Work out the finished part from the listing and answer in its coordinate system (mm). A direction names the side the tool comes from. Give positions to 0.01 mm unless a question says otherwise; leave off trailing zeros. Write each loop counter-clockwise with the first axis right and the second up, starting at its lowest first coordinate (ties: lowest second). Pieces come first, ordered by that corner, then holes.
1) Find section A-A (z = 43.5). Determine the outline of the cut face in (x, y).
2) Straight lines are drawn through the part: probe 1 along Y at (x, z) = (6.5, 62.5); probe 2 along Z at (x, y) = (12, 43); probe 3 along X at (y, z) = (4, 28.5). For each, find the intervals that lie inside material, in ascending order.
3) Find section B-B (y = 3.5). Determine the outline of the cut face in (x, z), plus the area to 3 significant figures.
4) Find section C-C (z = 30). Determine the outline of the cut face in (x, y).
5) Given pin 1 Ø1 at (x, z) = (-15, 25.5) entering from +Y; pin 2 Ø1 at (y, z) = (49.5, 27.5) entering from +X; pin 3 Ø1.1 at (y, z) = (48, 24) entering from +X, each flat-ended and moving along its own axis, determine where each tip first touches the part or whether it passes through.
6) A tool of negligible diameter and unlimited length cuts with its end or side. For faces 1 (the face through (62.568, 25, 32)), 2 (the face through (34, 15, 2)), 3 (the face through (-40, 36.036, 32)), 4 (the face through (11, 8, 62.296)), from which of +Z, -Z, +X, -X, +Y, -Y can it reach the whole face along a straight path? Write none if from no direction.
7) Find section D-D (x = 23). Determine the outline of the cut face in (y, z).
8) Determine the mould class of faces 5 (the face through (-40, 39, 37.296)), 6 (the face through (10, 25, 0.296)), 7 (the face through (34, 47.4, 2)), 8 (the face through (10, 2, 32)) for opening direction Y: pulls with the +Y half, pulls with the -Y half, needs draft (parallel to the pull), parting line crosses it, or undercut.
Autodesk Fusion 360 part; units mm, degrees
sketch "Esquisse1" plane through (0, 0, 0) normal (0, 1, 0) x (1, 0, 0)
  line L0 (-41.4317, -0.2961) -> (62.5683, -0.2961)
  line L1 (62.5683, -0.2961) -> (62.5683, -64.2961)
  line L2 (62.5683, -64.2961) -> (-41.4317, -64.2961)
  line L3 (-41.4317, -64.2961) -> (-41.4317, -0.2961)
  dimension "d1" = 104
  dimension "d2" = 64
extrude "Extrusion1" add sketch "Esquisse1" along normal blind 50
shell "Coque1" thickness 2 removed faces 1 at (-6.765, 50, 21.6294)
sketch "Sketch4" plane through (62.5683, 0, 0) normal (1, 0, 0) x (0, 1, 0)
  line L0 (0, 64.2961) -> (0, 0.2961)
  line L1 (0, 0.2961) -> (50, 0.2961)
  line L2 (50, 0.2961) -> (50, 64.2961)
  line L3 (50, 64.2961) -> (0, 64.2961)
  line L4 (0, 32.2961) -> (50, 32.2961) construction
  line L5 (15, 63.3961) -> (16.4, 63.3961)
  line L6 (16.4, 63.3961) -> (16.4, 1.1961)
  line L7 (16.4, 1.1961) -> (15, 1.1961)
  line L8 (15, 1.1961) -> (15, 63.3961)
  line L9 (48.8, 1.1961) -> (47.4, 1.1961)
  line L10 (47.4, 1.1961) -> (47.4, 63.3961)
  line L11 (47.4, 63.3961) -> (48.8, 63.3961)
  line L12 (48.8, 63.3961) -> (48.8, 1.1961)
  line L13 (48.8, 62.2961) -> (50, 62.2961)
  line L14 (48.8, 2.2961) -> (50, 2.2961)
  dimension "d19" = 1.4
  dimension "d20" = 1.4
  dimension "d55" = 31
  dimension "d66" = 0.9
  dimension "d67" = 2
  dimension "d79" = 15
extrude "Extrude4" cut sketch "Sketch4" against normal blind 103.1 contours L9 L10 L11 L12 | L5 L6 L7 L8
sketch "Sketch8" plane through (0, 50, 0) normal (0, 1, 0) x (-1, 0, 0)
  line L0 (39.4317, 2.2961) -> (-60.5683, 2.2961)
  line L1 (-60.5683, 62.2961) -> (39.4317, 62.2961)
  line L2 (41.4317, 64.2961) -> (-62.5683, 64.2961)
  line L3 (-62.5683, 64.2961) -> (-62.5683, 0.2961)
  line L4 (-62.5683, 0.2961) -> (41.4317, 0.2961)
  line L5 (41.4317, 0.2961) -> (41.4317, 64.2961)
  line L6 (-60.5683, 2.2961) -> (-62.5683, 2.2961)
  line L7 (-62.5683, 2.2961) -> (-62.5683, 42.2961)
  line L8 (-60.5683, 42.2961) -> (-60.5683, 2.2961)
  line L9 (39.4317, 62.2961) -> (39.4317, 2.2961)
  line L10 (-60.5683, 2.2961) -> (-60.5683, 62.2961)
  line L11 (-60.5683, 62.2961) -> (-62.5683, 62.2961)
  line L12 (-60.5683, 42.2961) -> (-60.5683, 62.2961)
  line L13 (-62.5683, 42.2961) -> (-62.5683, 2.2961)
extrude "Extrude6" cut sketch "Sketch8" against normal blind 1.3 contours L3 L6 L7 L8 L10 L11 L12 L13
sketch "Sketch9" plane through (0, 0, 64.2961) normal (0, 0, 1) x (-1, 0, 0)
  line L0 (-62.5683, 0) -> (-62.5683, -50)
  line L1 (-62.5683, -50) -> (41.4317, -50)
  line L2 (41.4317, -50) -> (41.4317, 0)
  line L3 (-62.5683, -45.1) -> (41.4317, -45.1) construction
  line L4 (-18.0683, -43.6) -> (-3.0683, -43.6)
  line L5 (-3.0683, -43.6) -> (-3.0683, -46.6)
  line L6 (-3.0683, -46.6) -> (-18.0683, -46.6)
  line L7 (-18.0683, -46.6) -> (-18.0683, -43.6)
  line L8 (-10.5683, -50) -> (-10.5683, -31.2) construction
  line L9 (41.4317, 0) -> (-62.5683, 0)
  dimension "d61" = 4.9
  dimension "d62" = 15
  dimension "d63" = 3
fillet "Fillet1" radius 1 4 edges at (10.5683, 0, 64.2961) (62.5683, 0, 32.2961) (10.5683, 0, 0.2961) (-41.4317, 0, 32.2961)
sketch "Sketch12" plane through (-41.4317, 0, 0) normal (-1, 0, 0) x (0, -1, 0)
  line L0 (-1, 0.2961) -> (-1, 64.2961)
  line L1 (-1, 64.2961) -> (-50, 64.2961)
  line L2 (-50, 64.2961) -> (-50, 0.2961)
  line L3 (-50, 0.2961) -> (-1, 0.2961)
  line L4 (-41.0361, 37.2961) -> (-36.0361, 37.2961)
  line L5 (-36.0361, 37.2961) -> (-36.0361, 27.2961)
  line L6 (-36.0361, 27.2961) -> (-41.0361, 27.2961)
  line L7 (-41.0361, 27.2961) -> (-41.0361, 37.2961)
  line L8 (-1, 32.2961) -> (-50, 32.2961) construction
  dimension "d80" = 5
  dimension "d81" = 10
extrude "Extrude10" cut sketch "Sketch12" against normal blind 15 contours L4 L5 L6 L7
Results:
1. outline: (-41.43, 1) arc R1 ccw to (-40.43, 0) - (61.57, 0) arc R1 ccw to (62.57, 1) - (62.57, 15) - (60.57, 15) - (60.57, 2) - (-39.43, 2) - (-39.43, 15) - (-40.53, 15) - (-40.53, 16.4) - (-39.43, 16.4) - (-39.43, 47.4) - (-40.53, 47.4) - (-40.53, 48.8) - (-39.43, 48.8) - (-39.43, 50) - (-41.43, 50) - close; (60.57, 16.4) - (62.57, 16.4) - (62.57, 47.4) - (60.57, 47.4) - close
2. probe 1: y = 0 to 15, 16.4 to 47.4, 48.8 to 50
2. probe 2: z = 0.3 to 2.3, 62.3 to 64.3
2. probe 3: x = -41.43 to -39.43, 60.57 to 62.57
3. outline: (-41.43, 0.3) - (62.57, 0.3) - (62.57, 64.3) - (-41.43, 64.3) - close; hole (-39.43, 2.3) - (60.57, 2.3) - (60.57, 62.3) - (-39.43, 62.3) - close
3. area: 656 mm2
4. outline: (-41.43, 1) arc R1 ccw to (-40.43, 0) - (61.57, 0) arc R1 ccw to (62.57, 1) - (62.57, 15) - (60.57, 15) - (60.57, 2) - (-39.43, 2) - (-39.43, 15) - (-40.53, 15) - (-40.53, 16.4) - (-39.43, 16.4) - (-39.43, 36.04) - (-41.43, 36.04) - close; (-41.43, 41.04) - (-39.43, 41.04) - (-39.43, 47.4) - (-40.53, 47.4) - (-40.53, 48.8) - (-39.43, 48.8) - (-39.43, 50) - (-41.43, 50) - close; (60.57, 16.4) - (62.57, 16.4) - (62.57, 47.4) - (60.57, 47.4) - close
5. pin 1: stops at y = 2
5. pin 2: stops at x = -39.43
5. pin 3: stops at x = -40.53
6. face 1: +Z, -Z, +X, +Y, -Y
6. face 2: +X
6. face 3: -X
6. face 4: +Y
7. outline: (0, 1.3) arc R1 ccw to (1, 0.3) - (50, 0.3) - (50, 2.3) - (48.8, 2.3) - (48.8, 1.2) - (47.4, 1.2) - (47.4, 2.3) - (16.4, 2.3) - (16.4, 1.2) - (15, 1.2) - (15, 2.3) - (2, 2.3) - (2, 62.3) - (15, 62.3) - (15, 63.4) - (16.4, 63.4) - (16.4, 62.3) - (47.4, 62.3) - (47.4, 63.4) - (48.8, 63.4) - (48.8, 62.3) - (50, 62.3) - (50, 64.3) - (1, 64.3) arc R1 ccw to (0, 63.3) - close
8. face 5: undercut
8. face 6: needs draft
8. face 7: undercut
8. face 8: pulls with the +Y half
